Can you work these out from the model? Positions are in its coordinate system, mm. A direction names the side the tool comes from. Give positions to 0.01 mm unless a question says otherwise; leave off trailing zeros. Order: outer loops, then holes, each group sorted by start corner. A loop starts at its lowest first (then second) coordinate and runs counter-clockwise, first axis right, second up. Notation, with made-up numbers: M -2,21.25 L 9,21.25 A10 cw 9,36.25 Z; hole C 49,78.25 d7. An arc over 180 degrees is marked long. Use one line per item in the form item = value. Start each with the question number.
1. I want a section at A-A, the plane z = 30. List the corners of the cut face in (x, y) for me.
2. I want a section at C-C, the plane x = 42. List the corners of the cut face in (y, z) for me.
3. I want a section at B-B, the plane y = 0.75. List the corners of the cut face in (x, z) for me, and give its area (3 significant figures).
4. We'd pull the mould along Z, two halves only. Please class faces 1 (the face through (-23.993, 1.014, -10.924)), 2 (the face through (60, 2, -30)), 3 (the face through (-57.15, 2.54, 56.99)): +Z half, -Z half, draft (parallel to the pull), parting line (faces both ways), or undercut.
5. For faces 4 (the face through (-44, 2, -15)), 5 (the face through (60, 3, 30)), 6 (the face through (85, 3, -10)), 7 (the face through (-85, 3, -10)), which set-ups out of +Z, -Z, +X, -X, +Y, -Y let a thin tool reach every point of the face, with its end or its side?
6. Will these pins go through, and if not, where does the flat tip stop? P1, Ø1.5, axis at y = 3, z = -58.5, coming from the -X side; P2, Ø1, axis at y = 2.5, z = -41, coming from the -X side; P3, Ø1.5, axis at x = 73, y = 1.5, coming from the +Z side.
7. I want a section at D-D, the plane z = -5.5. List the corners of the cut face in (x, y) for me.
8. I need wall thicknesses on L1, parallel to X at y = 2.4, z = 47.5; L2, parallel to X at y = 4.35, z = 36; L3, parallel to Z at x = 87, y = 0.3. Which ranges of each line are inside material? Lowest first, please.
```python
from build123d import *

# Parameters (mm, degrees)
SKETCH1_W           = 120
SKETCH1_H           = 120
BOSS_EXTRUDE1_DEPTH = 5
SKETCH2_R           = 20
CUT_EXTRUDE4_DEPTH  = 5
SKETCH3_R           = 26.6
SKETCH3_R_2         = 20
CUT_EXTRUDE5_DEPTH  = 3
SKETCH4_W           = 60
SKETCH4_H           = 5
BOSS_EXTRUDE2_DEPTH = 50
SKETCH5_W           = 60
SKETCH5_H           = 5
BOSS_EXTRUDE3_DEPTH = 50
FILLET3_R           = 10
FILLET4_R           = 10
FILLET5_R           = 10
FILLET6_R           = 10
SKETCH8_W           = 50
SKETCH8_H           = 20
CUT_EXTRUDE6_DEPTH  = 10
SKETCH10_W          = 2.261137553
SKETCH10_H          = 2.574285836
CUT_EXTRUDE7_DEPTH  = 2
SKETCH12_W          = 5.377639696
SKETCH12_H          = 6.736845814
CUT_EXTRUDE10_DEPTH = 3
SKETCH14_W          = 4.90266265
SKETCH14_H          = 7.042630192
CUT_EXTRUDE11_DEPTH = 3


with BuildPart() as part:
    # Sketch1 → Boss-Extrude1 (new body)
    with BuildSketch(Plane(origin=(0, 0, 0), x_dir=(1, 0, 0), z_dir=(0, 1, 0))):
        Rectangle(SKETCH1_W, SKETCH1_H)
    extrude(amount=BOSS_EXTRUDE1_DEPTH)

    # Sketch2 → Cut-Extrude4 (cut)
    with BuildSketch(Plane(origin=(0, 5, 0), x_dir=(1, 0, 0), z_dir=(0, 1, 0))):
        with Locations(Location((30, 30, 0), (0, 0, 270))):
            Circle(SKETCH2_R)
        with Locations(Location((-30, -30, 0), (0, 0, 270))):
            Circle(SKETCH2_R)
        with Locations(Location((30, -30, 0), (0, 0, 270))):
            Circle(SKETCH2_R)
        with Locations(Location((-30, 30, 0), (0, 0, 270))):
            Circle(SKETCH2_R)
    extrude(amount=-CUT_EXTRUDE4_DEPTH, mode=Mode.SUBTRACT)

    # Sketch3 → Cut-Extrude5 (cut)
    # profile 1 of 4: a face of its own
    with BuildSketch(Plane(origin=(0, 5, 0), x_dir=(1, 0, 0), z_dir=(0, 1, 0))):
        with Locations(Location((30, 30, 0), (0, 0, 270))):
            Circle(SKETCH3_R)
        with Locations(Location((30, 30, 0), (0, 0, 270))):
            Circle(SKETCH3_R_2, mode=Mode.SUBTRACT)
    # profile 2 of 4: a face of its own
    with BuildSketch(Plane(origin=(0, 5, 0), x_dir=(1, 0, 0), z_dir=(0, 1, 0))):
        with Locations(Location((-30, -30, 0), (0, 0, 270))):
            Circle(SKETCH3_R)
        with Locations(Location((-30, -30, 0), (0, 0, 270))):
            Circle(SKETCH3_R_2, mode=Mode.SUBTRACT)
    # profile 3 of 4: a face of its own
    with BuildSketch(Plane(origin=(0, 5, 0), x_dir=(1, 0, 0), z_dir=(0, 1, 0))):
        with Locations(Location((30, -30, 0), (0, 0, 270))):
            Circle(SKETCH3_R)
        with Locations(Location((30, -30, 0), (0, 0, 270))):
            Circle(SKETCH3_R_2, mode=Mode.SUBTRACT)
    # profile 4 of 4: a face of its own
    with BuildSketch(Plane(origin=(0, 5, 0), x_dir=(1, 0, 0), z_dir=(0, 1, 0))):
        with Locations(Location((-30, 30, 0), (0, 0, 270))):
            Circle(SKETCH3_R)
    extrude(amount=-CUT_EXTRUDE5_DEPTH, mode=Mode.SUBTRACT)

    # Sketch4 → Boss-Extrude2 (add)
    with BuildSketch(Plane(origin=(60, 0, 0), x_dir=(0, 0, -1), z_dir=(1, 0, 0))):
        with Locations((0, 2.5)):
            Rectangle(SKETCH4_W, SKETCH4_H)
    extrude(amount=BOSS_EXTRUDE2_DEPTH)

    # Sketch5 → Boss-Extrude3 (add)
    with BuildSketch(Plane.ZY.offset(60)):
        with Locations((0, 2.5)):
            Rectangle(SKETCH5_W, SKETCH5_H)
    extrude(amount=BOSS_EXTRUDE3_DEPTH)

    # Fillet3
    fillet3_edges = [part.edges().sort_by_distance(p)[0] for p in [
        (-60, 2.5, 60),
    ]]
    fillet(fillet3_edges, radius=FILLET3_R)

    # Fillet4
    fillet4_edges = [part.edges().sort_by_distance(p)[0] for p in [
        (60, 2.5, 60),
    ]]
    fillet(fillet4_edges, radius=FILLET4_R)

    # Fillet5
    fillet5_edges = [part.edges().sort_by_distance(p)[0] for p in [
        (-60, 2.5, -60),
    ]]
    fillet(fillet5_edges, radius=FILLET5_R)

    # Fillet6
    fillet6_edges = [part.edges().sort_by_distance(p)[0] for p in [
        (60, 2.5, -60),
    ]]
    fillet(fillet6_edges, radius=FILLET6_R)

    # Sketch8 → Cut-Extrude6 (cut)
    with BuildSketch(Plane(origin=(0, 5, 0), x_dir=(1, 0, 0), z_dir=(0, 1, 0))):
        with Locations((-85, 20)):
            Rectangle(SKETCH8_W, SKETCH8_H)
        with Locations((-85, -20)):
            Rectangle(SKETCH8_W, SKETCH8_H)
        with Locations((85, -20)):
            Rectangle(SKETCH8_W, SKETCH8_H)
        with Locations((85, 20)):
            Rectangle(SKETCH8_W, SKETCH8_H)
    extrude(amount=-CUT_EXTRUDE6_DEPTH, mode=Mode.SUBTRACT)

    # Sketch10 → Cut-Extrude7 (cut)
    with BuildSketch(Plane(origin=(0, 5, 0), x_dir=(1, 0, 0), z_dir=(0, 1, 0))):
        with Locations((-55.406362831, 0)):
            Rectangle(SKETCH10_W, SKETCH10_H)
    extrude(amount=-CUT_EXTRUDE7_DEPTH, mode=Mode.SUBTRACT)

    # Sketch12 → Cut-Extrude10 (cut)
    with BuildSketch(Plane(origin=(0, 5, 0), x_dir=(1, 0, 0), z_dir=(0, 1, 0))):
        with Locations((-30, -3.4)):
            Rectangle(SKETCH12_W, SKETCH12_H)
        with Locations((30, -3.4)):
            Rectangle(SKETCH12_W, SKETCH12_H)
    extrude(amount=-CUT_EXTRUDE10_DEPTH, mode=Mode.SUBTRACT)

    # Sketch14 → Cut-Extrude11 (cut)
    with BuildSketch(Plane(origin=(0, 5, 0), x_dir=(1, 0, 0), z_dir=(0, 1, 0))):
        with Locations((-30, 56.6)):
            Rectangle(SKETCH14_W, SKETCH14_H)
        with Locations((30, 56.6)):
            Rectangle(SKETCH14_W, SKETCH14_H)
    extrude(amount=-CUT_EXTRUDE11_DEPTH, mode=Mode.SUBTRACT)


solid = part.part
```
Check result:
q1.outline = M -60,0 L -50,0 L -50,2 L -56.6,2 L -56.6,5 L -60,5 Z; M -10,0 L 10,0 L 10,2 L 3.4,2 L 3.4,5 L -3.4,5 L -3.4,2 L -10,2 Z; M 50,0 L 60,0 L 60,5 L 56.6,5 L 56.6,2 L 50,2 Z
q2.outline = M 0,-60 L 5,-60 L 5,-53.74 L 2,-53.74 L 2,-46 L 0,-46 Z; M 0,-14 L 2,-14 L 2,-6.26 L 5,-6.26 L 5,6.26 L 2,6.26 L 2,14 L 0,14 Z; M 0,46 L 2,46 L 2,53.74 L 5,53.74 L 5,60 L 0,60 Z
q3.outline = M -110,-10 L -60,-10 L -60,-50 A10 ccw -50,-60 L 50,-60 A10 ccw 60,-50 L 60,-10 L 110,-10 L 110,10 L 60,10 L 60,50 A10 ccw 50,60 L -50,60 A10 ccw -60,50 L -60,10 L -110,10 Z; hole C -30,-30 d40; hole C -30,30 d40; hole C 30,-30 d40; hole C 30,30 d40
q3.area = 11,300 mm2
q4.face_1 = undercut
q4.face_2 = draft
q4.face_3 = +Z half
q5.face_4 = +Y
q5.face_5 = +Z, +X, +Y, -Y
q5.face_6 = -Z, +X, +Y, -Y
q5.face_7 = -Z, -X, +Y, -Y
q6.P1 = -56.32
q6.P2 = -60
q6.P3 = 10
q7.outline = M -110,0 L 110,0 L 110,5 L 40.36,5 L 40.36,2 L 19.64,2 L 19.64,5 L -19.64,5 L -19.64,2 L -40.36,2 L -40.36,5 L -110,5 Z
q8.L1 = -60 to -50.03, -9.97 to 9.97, 50.03 to 60
q8.L2 = -60 to -55.91, -4.09 to 4.09, 55.91 to 60
q8.L3 = -10 to 10
